```python
from build123d import *

# Parameters (mm, degrees)
BOSS_EXTRUDE1_DEPTH      = 39.6875
SKETCH3_R                = 1.5875
CUT_EXTRUDE1_DEPTH       = 39.6875
CUT_EXTRUDE3_DEPTH       = 5
CUT_EXTRUDE5_DEPTH       = 0.83
CUT_EXTRUDE5_DEPTH_BACK  = 5.67
FILLET1_R                = 0.508
SKETCH7_W                = 5.08
SKETCH7_H                = 10.72628101
BOSS_EXTRUDE2_DEPTH      = 1.905
SKETCH8_W                = 5.08
SKETCH8_H                = 3.15692897
BOSS_EXTRUDE3_DEPTH      = 10.16
CUT_EXTRUDE7_REACH       = 54.859
SKETCH9_R                = 1.05
FILLET2_R                = 0.381
CUT_EXTRUDE8_DEPTH       = 53.05177524
BOSS_EXTRUDE4_DEPTH      = 0.508
BOSS_EXTRUDE4_DEPTH_BACK = 39.1795
SKETCH11_W               = 3.175
SKETCH11_H               = 7.302
SKETCH11_W_2             = 4.84
SKETCH11_H_2             = 6.1
SKETCH11_W_3             = 5.720125627
SKETCH11_H_3             = 3.05
FILLET3_R                = 0.508
SKETCH13_W               = 4.84
SKETCH13_H               = 4.34094633
CUT_EXTRUDE10_DEPTH      = 3.048


with BuildPart() as part:
    # Sketch2 → Boss-Extrude1 (new body)
    with BuildSketch(Plane.XY):
        Polygon((-4.895, 3.02911179), (-9.97, 3.02911179), (-9.97, 10.33111179), (-2.42, 10.33111179), (-2.42, 7.28311179), (2.42, 7.28311179), (2.42, 10.33111179), (9.97, 10.33111179), (9.97, 3.02911179), (4.895, 3.02911179), (4.895, -1.82088821), (13.145, -1.82088821), (13.145, 13.37911179), (10.045, 13.37911179), (4.8375, 19.15761179), (4.8375, 22.33261179), (3.25, 22.33261179), (3.25, 21.57061179), (-3.25, 21.57061179), (-3.25, 22.33261179), (-4.8375, 22.33261179), (-4.8375, 19.15761179), (-10.045, 13.37911179), (-13.145, 13.37911179), (-13.145, -1.82088821), (-4.895, -1.82088821), align=None)
    extrude(amount=BOSS_EXTRUDE1_DEPTH)

    # Sketch3 → Cut-Extrude1 (cut)
    with BuildSketch(Plane(origin=(0, 21.57061179, 0), x_dir=(1, 0, 0), z_dir=(0, 1, 0))):
        with Locations(Location((0, -19.84375, 0), (0, 0, 270))):
            Circle(SKETCH3_R)
    extrude(amount=-CUT_EXTRUDE1_DEPTH, mode=Mode.SUBTRACT)

    # Sketch4 → Cut-Extrude3 (cut)
    with BuildSketch(Plane.XZ.offset(-7.28311179)):
        Polygon((1.760918321, 16.79375), (3.521836642, 19.84375), (1.760918321, 22.89375), (-1.760918321, 22.89375), (-3.521836642, 19.84375), (-1.760918321, 16.79375), align=None)
    extrude(amount=-CUT_EXTRUDE3_DEPTH, mode=Mode.SUBTRACT)

    # Sketch5 → Cut-Extrude5 (cut, two sides: drawn at the far end of the back side and taken through both)
    with BuildSketch(Plane.ZY.offset(2.42).offset(-CUT_EXTRUDE5_DEPTH_BACK)):
        with BuildLine():
            Line((21.966982917, 7.15761179), (21.966982917, 19.15761179))
            Line((21.966982917, 19.15761179), (23.966982917, 21.15761179))
            Line((23.966982917, 21.15761179), (15.626036587, 21.15761179))
            Line((15.626036587, 21.15761179), (17.626036587, 19.15761179))
            Line((17.626036587, 19.15761179), (17.626036587, 7.15761179))
            Line((17.626036587, 7.15761179), (9.473965766, 7.15761179))
            ThreePointArc((9.473965766, 7.15761179), (14.101249798, 15.593648004), (6.752192324, 21.804108435))
            Line((6.752192324, 21.804108435), (30.939378373, 21.804108435))
            ThreePointArc((30.939378373, 21.804108435), (24.928421122, 14.794550832), (30.119053738, 7.15761179))
            Line((30.119053738, 7.15761179), (21.966982917, 7.15761179))
        make_face()
    extrude(amount=CUT_EXTRUDE5_DEPTH + CUT_EXTRUDE5_DEPTH_BACK, mode=Mode.SUBTRACT)

    # Fillet1
    fillet1_edges = [part.edges().sort_by_distance(p)[0] for p in [
        (-13.145, 5.77911179, 39.6875),
        (-9.02, -1.82088821, 39.6875),
        (-9.97, 6.68011179, 39.6875),
        (-6.195, 10.33111179, 39.6875),
        (-2.42, 8.80711179, 39.6875),
        (-9.02, -1.82088821, 0),
        (0, 7.28311179, 39.6875),
        (-13.145, 5.77911179, 0),
        (-11.595, 13.37911179, 0),
        (-7.44125, 16.26836179, 0),
        (-4.8375, 20.74511179, 0),
        (-4.04375, 22.33261179, 0),
        (-3.25, 21.95161179, 0),
        (0, 21.57061179, 0),
        (3.25, 21.95161179, 0),
        (4.04375, 22.33261179, 0),
        (4.8375, 20.74511179, 0),
        (2.42, 8.80711179, 39.6875),
        (7.44125, 16.26836179, 0),
        (11.595, 13.37911179, 0),
        (13.145, 5.77911179, 0),
        (9.02, -1.82088821, 0),
        (4.895, 0.60411179, 0),
        (7.4325, 3.02911179, 0),
        (9.97, 6.68011179, 0),
        (6.195, 10.33111179, 0),
        (2.42, 8.80711179, 0),
        (0, 7.28311179, 0),
        (6.195, 10.33111179, 39.6875),
        (-2.42, 8.80711179, 0),
        (-6.195, 10.33111179, 0),
        (-9.97, 6.68011179, 0),
        (-7.4325, 3.02911179, 0),
        (-4.895, 0.60411179, 0),
        (9.97, 6.68011179, 39.6875),
        (7.4325, 3.02911179, 39.6875),
        (4.895, 0.60411179, 39.6875),
        (9.02, -1.82088821, 39.6875),
        (-4.895, 0.60411179, 39.6875),
        (13.145, 5.77911179, 39.6875),
        (11.595, 13.37911179, 39.6875),
        (7.44125, 16.26836179, 39.6875),
        (4.8375, 20.74511179, 39.6875),
        (4.04375, 22.33261179, 39.6875),
        (3.25, 21.95161179, 39.6875),
        (0, 21.57061179, 39.6875),
        (-3.25, 21.95161179, 39.6875),
        (-4.04375, 22.33261179, 39.6875),
        (-4.8375, 20.74511179, 39.6875),
        (-7.4325, 3.02911179, 39.6875),
        (-7.44125, 16.26836179, 39.6875),
        (-11.595, 13.37911179, 39.6875),
    ]]
    fillet(fillet1_edges, radius=FILLET1_R)

    # Sketch7 → Boss-Extrude2 (add)
    with BuildSketch(Plane(origin=(13.145, 0, 0), x_dir=(0, 0, -1), z_dir=(1, 0, 0))):
        with Locations((-36.6395, 3.542252295)):
            Rectangle(SKETCH7_W, SKETCH7_H)
        with Locations((-7.4295, 3.542252295)):
            Rectangle(SKETCH7_W, SKETCH7_H)
    extrude(amount=BOSS_EXTRUDE2_DEPTH)

    # Sketch8 → Boss-Extrude3 (add)
    with BuildSketch(Plane(origin=(15.05, 0, 0), x_dir=(0, 0, -1), z_dir=(1, 0, 0))):
        with Locations((-36.6395, -0.242423725)):
            Rectangle(SKETCH8_W, SKETCH8_H)
        with Locations((-7.4295, -0.242423725)):
            Rectangle(SKETCH8_W, SKETCH8_H)
    extrude(amount=BOSS_EXTRUDE3_DEPTH)

    # Sketch9 → Cut-Extrude7 (cut, up to next)
    with BuildSketch(Plane.XZ.offset(1.82088821), mode=Mode.PRIVATE) as cut_extrude7_sk1:
        with Locations((19.241, 35.8775)):
            Circle(SKETCH9_R)
    cut_extrude7_tool1 = extrude(cut_extrude7_sk1.sketch, amount=-CUT_EXTRUDE7_REACH, mode=Mode.PRIVATE) & part.part
    # Sketch9 → Cut-Extrude7 (cut, up to next)
    with BuildSketch(Plane.XZ.offset(1.82088821), mode=Mode.PRIVATE) as cut_extrude7_sk2:
        with Locations((19.241, 7.6835)):
            Circle(SKETCH9_R)
    cut_extrude7_tool2 = extrude(cut_extrude7_sk2.sketch, amount=-CUT_EXTRUDE7_REACH, mode=Mode.PRIVATE) & part.part
    add(cut_extrude7_tool1.solids().sort_by_distance((19.241, -1.820888, 35.8775))[0], mode=Mode.SUBTRACT)
    add(cut_extrude7_tool2.solids().sort_by_distance((19.241, -1.820888, 7.6835))[0], mode=Mode.SUBTRACT)

    # Fillet2
    fillet2_edges = [part.edges().sort_by_distance(p)[0] for p in [
        (18.191, 1.33604076, 35.8775),
        (18.191, -1.82088821, 35.8775),
        (18.191, 1.33604076, 7.6835),
        (18.191, -1.82088821, 7.6835),
    ]]
    fillet(fillet2_edges, radius=FILLET2_R)

    # Sketch10 → Cut-Extrude8 (cut, through all)
    with BuildSketch(Plane.XY.offset(39.6875)):
        Polygon((-8.140125627, 16.556662615), (-13.795, 16.556662615), (-15.501836838, 16.556662615), (-15.501836838, 5.924292452), (-8.140125627, 5.924292452), align=None)
        Polygon((-4.124785379, 5.924292452), (-8.140125627, 5.924292452), (-15.501836838, 5.924292452), (-15.501836838, -4.367210951), (-4.124785379, -4.367210951), align=None)
    extrude(amount=-CUT_EXTRUDE8_DEPTH, mode=Mode.SUBTRACT)

    # Sketch11 → Boss-Extrude4 (add, two sides: drawn at the far end of the back side and taken through both)
    with BuildSketch(Plane.XY.offset(39.1795).offset(-BOSS_EXTRUDE4_DEPTH_BACK)):
        with Locations((11.5575, -5.47188821)):
            Rectangle(SKETCH11_W, SKETCH11_H)
        with Locations((0, -9.12288821)):
            Rectangle(SKETCH11_W_2, SKETCH11_H_2)
        with Locations((-5.280062813, -10.64788821)):
            Rectangle(SKETCH11_W_3, SKETCH11_H_3)
    extrude(amount=BOSS_EXTRUDE4_DEPTH + BOSS_EXTRUDE4_DEPTH_BACK)


with BuildPart() as boss_extrude4_kept_piece:
    # of the separate pieces the step leaves, the one the design keeps (boss_extrude4_pieces_kept)
    add(part.part.solids().sort_by_distance((4.895, -1.82088821, 0.508))[0])

    # Fillet3
    fillet3_edges = [boss_extrude4_kept_piece.edges().sort_by_distance(p)[0] for p in [
        (11.5575, -9.12288821, 39.6875),
        (9.97, -9.12288821, 19.84375),
        (11.5575, -9.12288821, 0),
        (9.97, -5.47188821, 0),
        (13.145, -5.47188821, 0),
        (13.145, -5.47188821, 39.6875),
        (9.97, -5.47188821, 39.6875),
        (11.5575, -1.82088821, 39.6875),
        (11.5575, -1.82088821, 0),
    ]]
    fillet(fillet3_edges, radius=FILLET3_R - 0.0001)  # a hair under: the kernel refuses the full size

    # Sketch13 → Cut-Extrude10 (cut)
    with BuildSketch(Plane.XZ.offset(-7.28311179)):
        with Locations((0, 19.796509752)):
            Rectangle(SKETCH13_W, SKETCH13_H)
    extrude(amount=-CUT_EXTRUDE10_DEPTH, mode=Mode.SUBTRACT)


solid = boss_extrude4_kept_piece.part
```
Could you check a few things on this model? Use its own coordinates, in mm. A direction names the side the tool comes from. Coordinates: 2 decimals unless noted, no trailing zeros. Loops run counter-clockwise (first coordinate to the right, second up) from the corner with the lowest first, then second, coordinate; pieces in that order, holes last. Notation, with made-up numbers: M -6,21 L 13,21 A23 ccw 13,51 Z; hole C -9.75,-32.75 d5. An arc over 180 degrees is marked long. Put each result on its own line as item: value. Start each with the question number.
(1) Suppose I cut it at D-D on y = -3. Please give me the cut outline in (x, z) (1 decimal), then the cut area to 3 significant figures.
(2) Suppose I cut it at A-A on x = 0. Please give me the cut outline in (y, z).
(3) Suppose I cut it at B-B on x = 16.5. Please give me the cut outline in (y, z), then the cut area to 3 significant figures.
(4) For faces 1 (the face through (2.42, 9, 33)), 2 (the face through (18, 1, 34.1)), 3 (the face through (17.8, -1.821, 6.9)), 4 (the face through (-2.42, 9, 7)), 5 (the face through (0.05, 20.14, 22.95)), which set-ups out of +Z, -Z, +X, -X, +Y, -Y let a thin tool reach every point of the face, with its end or its side?
(5) Will these pins go through, and if not, where does the flat tip stop? P1, Ø3, axis at x = 1.5, z = 13.5, coming from the -Y side; P2, Ø2, axis at y = 14.5, z = 14, coming from the +X side; P3, Ø8, axis at y = 6, z = 10.5, coming from the -X side; P4, Ø1.5, axis at x = 14.5, z = 18, coming from the -Y side.
(6) Thinking about a two-plate mould opening in Z: for faces 6 (the face through (7.3, 16.197, 0.145)), 7 (the face through (0.046, 14.668, 24.922)), 8 (the face through (12, 13.379, 20)), 9 (the face through (12, -5, 39.688)), which applies, pulls with the +Z half, pulls with the -Z half, needs draft (parallel to the pull), parting line crosses it, or undercut?
(7) I need wall thicknesses on line 1 (X direction, y = 20, z = 2); line 2 (X direction, y = 5, z = 19) (3 decimals); line 3 (Y direction, x = -4.5, z = 37). Which ranges of each line are inside material? Lowest first, please. Write a range as from..to.
Solutions:
1. outline: M 10,0.5 A0.5 ccw 10.5,0 L 12.6,0 A0.5 ccw 13.1,0.5 L 13.1,39.2 A0.5 ccw 12.6,39.7 L 10.5,39.7 A0.5 ccw 10,39.2 Z
1. area: 126 mm2
2. outline: M 7.28,0.51 A0.51 ccw 7.79,0 L 21.06,0 A0.51 ccw 21.57,0.51 L 21.57,8.5 A7.6 ccw 7.28,9.77 Z; M 7.28,29.77 A7.6 ccw 21.57,30.09 L 21.57,39.18 A0.51 ccw 21.06,39.69 L 7.79,39.69 A0.51 ccw 7.28,39.18 Z; M 12.28,17.63 L 19.16,17.63 L 21.16,15.63 L 21.16,18.26 L 12.28,18.26 Z; M 12.28,21.43 L 21.16,21.43 L 21.16,23.97 L 19.16,21.97 L 12.28,21.97 Z
3. outline: M -1.82,4.89 L 1.34,4.89 L 1.34,9.97 L -1.82,9.97 Z; M -1.82,34.1 L 1.34,34.1 L 1.34,39.18 L -1.82,39.18 Z
3. area: 32.1 mm2
4. face 1: +Z, -Z, -Y
4. face 2: +X, +Y, -Y
4. face 3: +Z, -Z, +X, -Y
4. face 4: +Z, -Z, -X, -Y
4. face 5: -Y
5. P1: stops at y = 8.83
5. P2: stops at x = 9.94
5. P3: stops at x = -2.42
5. P4: passes through
6. face 6: pulls with the -Z half
6. face 7: undercut
6. face 8: needs draft
6. face 9: pulls with the +Z half
7. line 1: x = -4.84..4.84
7. line 2: x = 9.97..13.145
7. line 3: y = 10.33..22.33
